```python
from build123d import *

# Parameters (mm, degrees)
CROQUIS1_W              = 42
CROQUIS1_H              = 65
CROQUIS1_R              = 2.05
SALIENTE_EXTRUIR1_DEPTH = 4
CHAFL_N1_SIZE           = 4.1
CROQUIS5_R              = 5
CORTAR_EXTRUIR2_DEPTH   = 5


with BuildPart() as part:
    # Croquis1 → Saliente-Extruir1 (new body)
    with BuildSketch(Plane.XY):
        with Locations((21, 32.5)):
            Rectangle(CROQUIS1_W, CROQUIS1_H)
        with Locations((11, 56.8)):
            Circle(CROQUIS1_R, mode=Mode.SUBTRACT)
        with Locations((31, 56.8)):
            Circle(CROQUIS1_R, mode=Mode.SUBTRACT)
    extrude(amount=SALIENTE_EXTRUIR1_DEPTH)

    # Chaflán1
    chafl_n1_edges = [part.edges().sort_by_distance(p)[0] for p in [
        (42, 0, 2),
        (0, 0, 2),
    ]]
    chamfer(chafl_n1_edges, length=CHAFL_N1_SIZE)

    # Croquis5 → Cortar-Extruir2 (cut, through all)
    with BuildSketch(Plane.XY.offset(4)):
        with Locations((21, 21.08)):
            Circle(CROQUIS5_R)
    extrude(amount=-CORTAR_EXTRUIR2_DEPTH, mode=Mode.SUBTRACT)


solid = part.part
```
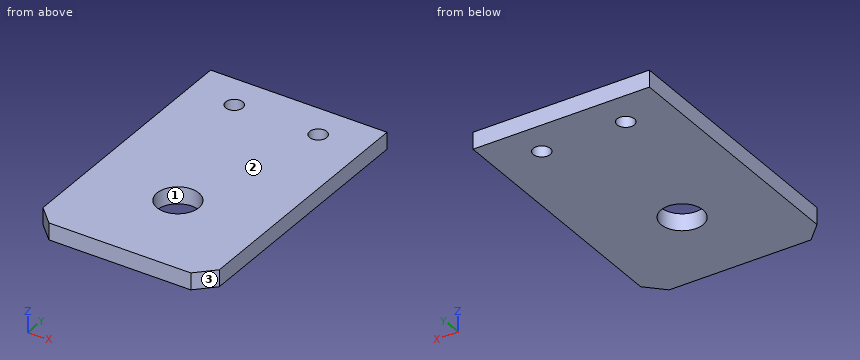
Check sheet for the modelled part. Datum: model origin and axes. Units: mm. Face numbers are marked on the shaded views. Give positions to 0.01 mm unless a question says otherwise; leave off trailing zeros. Loops run counter-clockwise (first coordinate to the right, second up) from the corner with the lowest first, then second, coordinate; pieces in that order, holes last. Notation, with made-up numbers: M 82,58.25 L 92,58.25 A10 cw 92,64.25 Z; hole C 72.5,-5.5 d9. An arc over 180 degrees is marked long. Answer as CSV lines item,"result".
Item 1: Depth check by flat-ended pin: pin 1 Ø3.5 at (x, y) = (11, 56.8) entering from -Z. Enter the tip coordinate at first touch or a pass-through.
Reply:
pin 1,"through"
Item 2: Sectioned sample at B-B, the plane y = 56.8. Enter the section's corners in (x, z), then the cut area to 3 significant figures.
Reply:
outline,"M 0,0 L 8.95,0 L 8.95,4 L 0,4 Z; M 13.05,0 L 28.95,0 L 28.95,4 L 13.05,4 Z; M 33.05,0 L 42,0 L 42,4 L 33.05,4 Z"
area,"135 mm^2"
Item 3: Sectioned sample at A-A, the plane x = 21. Enter the section's corners in (y, z).
Reply:
outline,"M 0,0 L 16.08,0 L 16.08,4 L 0,4 Z; M 26.08,0 L 65,0 L 65,4 L 26.08,4 Z"
Item 4: Sectioned sample at C-C, the plane z = 1.5. Enter the section's corners in (x, y).
Reply:
outline,"M 0,4.1 L 4.1,0 L 37.9,0 L 42,4.1 L 42,65 L 0,65 Z; hole C 11,56.8 d4.1; hole C 21,21.08 d10; hole C 31,56.8 d4.1"
Item 5: Sectioned sample at D-D, the plane x = 11. Enter the section's corners in (y, z), then the cut area to 3 significant figures.
Reply:
outline,"M 0,0 L 54.75,0 L 54.75,4 L 0,4 Z; M 58.85,0 L 65,0 L 65,4 L 58.85,4 Z"
area,"244 mm^2"
Item 6: Draft check along X on the marked faces 1, 2 and 3. Enter one of: pulls with the +X half, pulls with the -X half, needs draft (parallel to the pull), parting line crosses it, or undercut.
Reply:
face 1,"undercut"
face 2,"needs draft"
face 3,"pulls with the +X half"
Item 7: Scan lines: L1, parallel to Y at x = 31, z = 1.6; L2, parallel to X at y = 55.5, z = 3.5; L3, parallel to X at y = 21, z = 3.75. Record each from-to range of solid material in increasing order.
Reply:
L1,"0 to 54.75, 58.85 to 65"
L2,"0 to 9.41, 12.59 to 29.41, 32.59 to 42"
L3,"0 to 16, 26 to 42"
